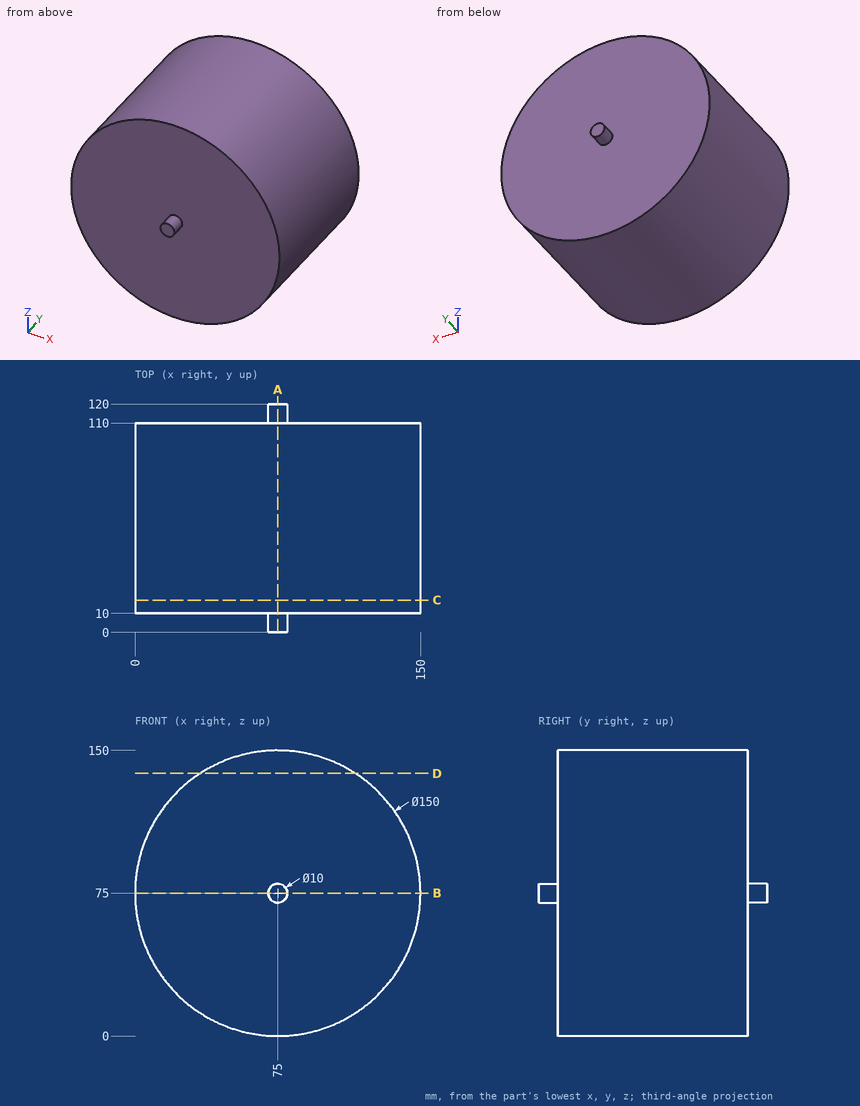
Can you work these out from the drawing? Everything is in mm from the part's minimum corner. Round coordinates to 2 decimals unless told otherwise and drop trailing zeros. Write each loop counter-clockwise with the first axis right and the second up, starting at its lowest first coordinate (ties: lowest second). Pieces come first, ordered by that corner, then holes.
1. I need wall thicknesses on L1, parallel to Y at x = 26, z = 92; L2, parallel to X at y = 62, z = 96; L3, parallel to X at y = 44.5, z = 143. Which ranges of each line are inside material? Lowest first, please.
2. Suppose I cut it at D-D (z = 138). List the corners of the cut face in (x, y) for me, and give its area (3 significant figures).
3. Suppose I cut it at C-C (y = 17). List the corners of the cut face in (x, z) for me, and give its area (3 significant figures).
4. Suppose I cut it at B-B (z = 75). List the corners of the cut face in (x, y) for me.
5. Will these pins go through, and if not, where does the flat tip stop? pin 1 Ø10 at (x, z) = (86, 49) entering from -Y; pin 2 Ø10 at (y, z) = (91, 92.5) entering from +X; pin 3 Ø8 at (x, y) = (67, 86) entering from -Z.
6. Suppose I cut it at A-A (x = 75). List the corners of the cut face in (y, z) for me, and give its area (3 significant figures).
Answer sheet:
1. L1: y = 10 to 110
1. L2: x = 3 to 147
1. L3: x = 43.36 to 106.64
2. outline: (34.31, 10) - (115.69, 10) - (115.69, 110) - (34.31, 110) - close
2. area: 8,140 mm2
3. outline: circle Ø150 at (75, 75)
3. area: 17,700 mm2
4. outline: (0, 10) - (70, 10) - (70, 0) - (80, 0) - (80, 10) - (150, 10) - (150, 110) - (80, 110) - (80, 120) - (70, 120) - (70, 110) - (0, 110) - close
5. pin 1: stops at y = 10
5. pin 2: stops at x = 148.95
5. pin 3: stops at z = 0.11
6. outline: (0, 70) - (10, 70) - (10, 0) - (110, 0) - (110, 70) - (120, 70) - (120, 80) - (110, 80) - (110, 150) - (10, 150) - (10, 80) - (0, 80) - close
6. area: 15,200 mm2
